Could you check a few things on this drawing? It's one solid part, dimensions in mm from its lowest x, y, z. A direction names the side the tool comes from. Give positions to 0.01 mm unless a question says otherwise; leave off trailing zeros. Write each loop counter-clockwise with the first axis right and the second up, starting at its lowest first coordinate (ties: lowest second). Pieces come first, ordered by that corner, then holes. Notation, with made-up numbers: M -11.5,-29 L 45.5,-29 A24 cw 45.5,-6 Z; hole C 4,-11.5 d9. An arc over 180 degrees is marked long. Write each question's results on one line, items separated by ' | '.
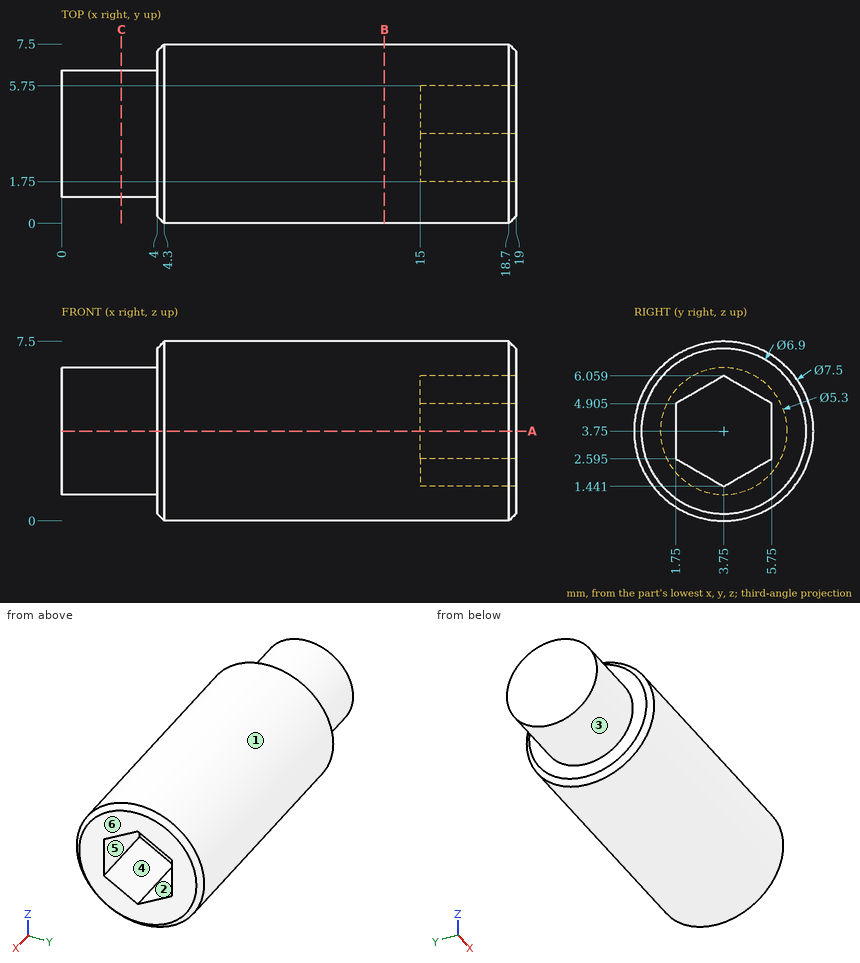
Item 1: Thinking about a two-plate mould opening in Z: for the marked faces 3, 4, 5 and 6, which applies, +Z half, -Z half, draft (parallel to the pull), parting line (faces both ways), or undercut?
Geometry says:
face 3: parting line | face 4: undercut | face 5: undercut | face 6: draft
Item 2: I'm going to push flat-ended pins straight in: pin 1 (1.2 mm diameter, centred on x = 18, z = 3.5, fed in from -Y); pin 2 (1 mm diameter, centred on x = 10.5, z = 6.5, fed in from -Y); pin 3 (3 mm diameter, centred on x = 7.5, z = 1, fed in from -Y) (1 decimal); pin 4 (1.2 mm diameter, centred on y = 4, z = 3, fed in from +X). Where does each tip first touch, or does it pass through?
Geometry says:
pin 1: stops at y = 0 | pin 2: stops at y = 0.75 | pin 3: stops at y = 0.2 | pin 4: stops at x = 15
Item 3: I want a section at C-C, the plane x = 2.5. Please give me the cut outline in (y, z).
Geometry says:
outline: C 3.75,3.75 d5.3
Item 4: I want a section at B-B, the plane x = 13.5. Please give me the cut outline in (y, z), and give its area (3 significant figures).
Geometry says:
outline: C 3.75,3.75 d7.5 | area: 44.2 mm2
Item 5: If I drill on line 1 (X direction, y = 4.5, z = 2.5); line 2 (Z direction, x = 15.5, y = 2.5) (1 decimal); line 3 (Z direction, x = 15.25, y = 3) (1 decimal), over which ranges is the centre line in solid material (lowest first)? Write a range as from..to.
Geometry says:
line 1: x = 0..15 | line 2: z = 0.2..2.2, 5.3..7.3 | line 3: z = 0.1..1.9, 5.6..7.4
Item 6: I want a section at A-A, the plane z = 3.75. Please give me the cut outline in (x, y).
Geometry says:
outline: M 0,1.1 L 4,1.1 L 4,0.3 L 4.3,0 L 18.7,0 L 19,0.3 L 19,1.75 L 15,1.75 L 15,5.75 L 19,5.75 L 19,7.2 L 18.7,7.5 L 4.3,7.5 L 4,7.2 L 4,6.4 L 0,6.4 Z
Item 7: For the marked faces 1 and 2, which set-ups out of +Z, -Z, +X, -X, +Y, -Y let a thin tool reach every point of the face, with its end or its side?
Geometry says:
face 1: +X, -X | face 2: +X
